Can you work these out from the model? Positions are in its coordinate system, mm. A direction names the side the tool comes from. Coordinates: 2 decimals unless noted, no trailing zeros. Order: outer loops, then holes, each group sorted by start corner. A loop starts at its lowest first (then second) coordinate and runs counter-clockwise, first axis right, second up. Notation, with made-up numbers: (69, 85.25) -> (94, 85.25) arc R20 ccw to (94, 104.25) -> close; hole circle Ø10 at (75.5, 8). An arc over 180 degrees is marked (long way). Write item = value, one per line. Start each with the question number.
from build123d import *

# Parameters (mm, degrees)
F0_W     = 279.4
F0_H     = 228.6
F1_DEPTH = 2.286
F3_DEPTH = 2.287
F4_R     = 1.6256
F5_DEPTH = 2.287


with BuildPart() as f1:
    # F0 (on Top) → F1 (new body)
    with BuildSketch(Plane.XY):
        Rectangle(F0_W, F0_H)
    extrude(amount=F1_DEPTH)

    # F2 (on face) → F3 (cut, through all)
    with BuildSketch(Plane.XY.offset(2.286)):
        with BuildLine():
            Line((-170.557151, 110.44136), (-117.59327, 69.939569))
            ThreePointArc((-117.59327, 69.939569), (-95.339569, 72.90673), (-98.30673, 95.160431))
            Line((-98.30673, 95.160431), (-151.27061, 135.662221))
            Line((-151.27061, 135.662221), (-170.557151, 110.44136))
        make_face()
        with BuildLine():
            Line((151.27061, 135.662221), (98.30673, 95.160431))
            ThreePointArc((98.30673, 95.160431), (95.339569, 72.90673), (117.59327, 69.939569))
            Line((117.59327, 69.939569), (170.557151, 110.44136))
            Line((170.557151, 110.44136), (151.27061, 135.662221))
        make_face()
        with BuildLine():
            Line((170.557151, -110.44136), (117.59327, -69.939569))
            ThreePointArc((117.59327, -69.939569), (95.339569, -72.90673), (98.30673, -95.160431))
            Line((98.30673, -95.160431), (151.27061, -135.662221))
            Line((151.27061, -135.662221), (170.557151, -110.44136))
        make_face()
        with BuildLine():
            Line((-151.27061, -135.662221), (-98.30673, -95.160431))
            ThreePointArc((-98.30673, -95.160431), (-95.339569, -72.90673), (-117.59327, -69.939569))
            Line((-117.59327, -69.939569), (-170.557151, -110.44136))
            Line((-170.557151, -110.44136), (-151.27061, -135.662221))
        make_face()
    extrude(amount=-F3_DEPTH, mode=Mode.SUBTRACT)

    # F4 (on face) → F5 (cut, through all)
    with BuildSketch(Plane.XY.offset(2.286)):
        with Locations((76.2, 0)):
            Circle(F4_R)
        with Locations((-76.2, 0)):
            Circle(F4_R)
    extrude(amount=-F5_DEPTH, mode=Mode.SUBTRACT)


solid = f1.part
(1) For faces 3 (the face through (110.65, -104.6, 1.16)), 4 (the face through (-128.49, -78.27, 1.16)), 5 (the face through (-2, 2, 0)), 6 (the face through (-110.65, 104.6, 1.16)), which set-ups out of +Z, -Z, +X, -X, +Y, -Y let a thin tool reach every point of the face, with its end or its side?
(2) Imagine slicing it at C-C (x = -110). Write out the boundary of the cut face in (y, z).
(3) Imagine slicing it at B-B (y = 76). Write out the boundary of the cut face in (x, z).
(4) For P1, Ø2.5, axis at x = 76.2, y = 0, coming from the -Z side, with a flat end and sliding along its axis, tell me the tip position at first contact or that it passes through.
(5) Thinking about a two-plate mould opening in Y: for faces 1 (the face through (-128.8, 78.51, 1.16)), 2 (the face through (-2, 2, 2.286)), which applies, +Y half, -Y half, draft (parallel to the pull), parting line (faces both ways), or undercut?
(6) If I drill on L1, parallel to Y at x = 76.2, z = 1.25; L2, parallel to X at y = -68.5, z = 0.7; L3, parallel to X at y = -70, z = 0.5, over which ranges is the centre line in solid material (lowest first)? Write a range as from..to.
(7) Imagine slicing it at A-A (z = 0.75). Write out the boundary of the cut face in (x, y) (3 decimals), plus the area to 3 significant figures.
Result set:
q1.face_3 = +Z, -Z, +X
q1.face_4 = +Z, -Z
q1.face_5 = -Z, +X, -X, +Y, -Y
q1.face_6 = +Z, -Z, -X
q2.outline = (-114.3, 0) -> (-104.1, 0) -> (-104.1, 2.29) -> (-114.3, 2.29) -> close; (-66.81, 0) -> (66.81, 0) -> (66.81, 2.29) -> (-66.81, 2.29) -> close; (104.1, 0) -> (114.3, 0) -> (114.3, 2.29) -> (104.1, 2.29) -> close
q3.outline = (-139.7, 0) -> (-125.52, 0) -> (-125.52, 2.29) -> (-139.7, 2.29) -> close; (-93.49, 0) -> (93.49, 0) -> (93.49, 2.29) -> (-93.49, 2.29) -> close; (125.52, 0) -> (139.7, 0) -> (139.7, 2.29) -> (125.52, 2.29) -> close
q4.P1 = through
q5.face_1 = undercut
q5.face_2 = draft
q6.L1 = -114.3..-1.63, 1.63..114.3
q6.L2 = -139.7..-115.34, -100.56..100.56, 115.34..139.7
q6.L3 = -139.7..-117.67, -98.23..98.23, 117.67..139.7
q7.outline = (-139.7, -86.845) -> (-117.593, -69.94) arc R15.875 cw to (-98.307, -95.16) -> (-123.335, -114.3) -> (123.335, -114.3) -> (98.307, -95.16) arc R15.875 cw to (117.593, -69.94) -> (139.7, -86.845) -> (139.7, 86.845) -> (117.593, 69.94) arc R15.875 cw to (98.307, 95.16) -> (123.335, 114.3) -> (-123.335, 114.3) -> (-98.307, 95.16) arc R15.875 cw to (-117.593, 69.94) -> (-139.7, 86.845) -> close; hole circle Ø3.251 at (-76.2, 0); hole circle Ø3.251 at (76.2, 0)
q7.area = 57,600 mm2
